Can you work these out from the model? Positions are in its coordinate system, mm. Face numbers are marked on the shaded views. A direction names the side the tool comes from. Round coordinates to 2 decimals unless told otherwise and drop trailing zeros. Order: outer loops, then holes, each group sorted by start corner. A loop starts at its lowest first (then second) coordinate and runs counter-clockwise, first axis right, second up. Notation, with made-up numbers: M -21.75,44.25 L 10.25,44.25 A16 cw 10.25,48.25 Z; hole C 37,44 d7. An arc over 180 degrees is marked long. Answer as a JSON object with one key per item and string values. Group by question number.
from build123d import *

# Parameters (mm, degrees)
BOX013_W                   = 14
BOX013_H                   = 3
BOX013_DEPTH               = 18
CYLINDER006_R              = 3.5
CYLINDER006_DEPTH          = 8
CYLINDER006_ROLL_ANGLE     = -90
CYLINDER_R                 = 0.6
CYLINDER_DEPTH             = 11
PRISM_DEPTH                = 10
PRISM_ROLL_ANGLE           = 90.00003
PRISM_PITCH_ANGLE          = -30.000033
PRISM_PLACEMENT_ANGLE      = -8e-06
BOX001_W                   = 10
BOX001_H                   = 18
BOX001_DEPTH               = 20
BOX002_W                   = 10
BOX002_H                   = 11
BOX002_DEPTH               = 15
BOX003_W                   = 10
BOX003_H                   = 25
BOX003_DEPTH               = 12
BOX004_W                   = 8.5
BOX004_H                   = 4
BOX004_DEPTH               = 7
BOX005_W                   = 8
BOX005_H                   = 4
BOX005_DEPTH               = 10.5
BOX006_W                   = 8.5
BOX006_H                   = 4
BOX006_DEPTH               = 7
BOX007_W                   = 13
BOX007_H                   = 4
BOX007_DEPTH               = 8
BOX008_W                   = 10
BOX008_H                   = 8.5
BOX008_DEPTH               = 8
BOX009_W                   = 5
BOX009_H                   = 14
BOX009_DEPTH               = 9
BOX010_W                   = 43
BOX010_H                   = 4
BOX010_DEPTH               = 19
SKETCH075_R                = 1.4
EXTRUDE_DEPTH              = 12
BOX011_W                   = 14
BOX011_H                   = 4
BOX011_DEPTH               = 12
BOX_W                      = 10
BOX_H                      = 56.75
BOX_DEPTH                  = 12
EXTRUDE073_DEPTH           = 25
EXTRUDE072_DEPTH           = 25
SKETCH072_R                = 4
SKETCH072_R_2              = 1.4
SKETCH072_R_3              = 2.25
EXTRUDE071_DEPTH           = 22.4
BOX012_W                   = 13
BOX012_H                   = 3
BOX012_DEPTH               = 15
EXTRUDE080_DEPTH           = 2.5
SKETCH071_W                = 47
SKETCH071_H                = 15
EXTRUDE070_DEPTH           = 2
EXTRUDE070_ROLL_ANGLE      = -0.000172
EXTRUDE070_PITCH_ANGLE     = -0.040176
EXTRUDE070_PLACEMENT_ANGLE = 2.8e-05


with BuildPart() as cube013:
    # Box013 → Box013 (new body)
    with BuildSketch(Plane(origin=(8, -54.5, 7), x_dir=(1, 0, 0), z_dir=(0, 0, 1))):
        with Locations((7, 1.5)):
            Rectangle(BOX013_W, BOX013_H)
    extrude(amount=BOX013_DEPTH)


with BuildPart() as cylinder006:
    # Cylinder006 → Cylinder006 (new body)
    with BuildSketch(Plane.XY):
        Circle(CYLINDER006_R)
    extrude(amount=CYLINDER006_DEPTH)


with BuildPart() as cylinder006_1:
    # Cylinder006 roll: moved
    add(cylinder006.part.rotate(Axis((0, 0, 0), (1, 0, 0)), CYLINDER006_ROLL_ANGLE))


with BuildPart() as cylinder006_2:
    # Cylinder006 placement: moved
    add(cylinder006_1.part.moved(Location((42.4, 48, 10))))


with BuildPart() as cylinder:
    # Cylinder → Cylinder (new body)
    with BuildSketch(Plane(origin=(46.125, 51.85, 17), x_dir=(1, 0, 0), z_dir=(0, 0, 1))):
        Circle(CYLINDER_R)
    extrude(amount=CYLINDER_DEPTH)


with BuildPart() as fusion032:
    # Prism → Prism (new body)
    with BuildSketch(Plane.XY):
        Polygon((5, 0), (2.5, 4.330127), (-2.5, 4.330127), (-5, 0), (-2.5, -4.330127), (2.5, -4.330127), align=None)
    extrude(amount=PRISM_DEPTH)


with BuildPart() as fusion032_1:
    # Prism roll: moved
    add(fusion032.part.rotate(Axis((0, 0, 0), (1, 0, 0)), PRISM_ROLL_ANGLE))


with BuildPart() as fusion032_2:
    # Prism pitch: moved
    add(fusion032_1.part.rotate(Axis((0, 0, 0), (0, 1, 0)), PRISM_PITCH_ANGLE))


with BuildPart() as fusion032_3:
    # Prism placement: moved
    add(fusion032_2.part.moved(Location((42.4, 51.75, 10))).rotate(Axis((42.4, 51.75, 10), (0, 0, 1)), PRISM_PLACEMENT_ANGLE))

    # Fusion032: union Cylinder006, Cylinder
    add(cylinder006_2.part)
    add(cylinder.part)


with BuildPart() as cube001:
    # Box001 → Box001 (new body)
    with BuildSketch(Plane(origin=(-67, 15.5, 8.5), x_dir=(1, 0, 0), z_dir=(0, 0, 1))):
        with Locations((5, 9)):
            Rectangle(BOX001_W, BOX001_H)
    extrude(amount=BOX001_DEPTH)


with BuildPart() as cube002:
    # Box002 → Box002 (new body)
    with BuildSketch(Plane(origin=(54, -25, 12), x_dir=(1, 0, 0), z_dir=(0, 0, 1))):
        with Locations((5, 5.5)):
            Rectangle(BOX002_W, BOX002_H)
    extrude(amount=BOX002_DEPTH)


with BuildPart() as cube003:
    # Box003 → Box003 (new body)
    with BuildSketch(Plane(origin=(54, -14, 15), x_dir=(1, 0, 0), z_dir=(0, 0, 1))):
        with Locations((5, 12.5)):
            Rectangle(BOX003_W, BOX003_H)
    extrude(amount=BOX003_DEPTH)


with BuildPart() as cube004:
    # Box004 → Box004 (new body)
    with BuildSketch(Plane(origin=(32.75, 51, 20), x_dir=(1, 0, 0), z_dir=(0, 0, 1))):
        with Locations((4.25, 2)):
            Rectangle(BOX004_W, BOX004_H)
    extrude(amount=BOX004_DEPTH)


with BuildPart() as cube005:
    # Box005 → Box005 (new body)
    with BuildSketch(Plane(origin=(19, 51, 16.5), x_dir=(1, 0, 0), z_dir=(0, 0, 1))):
        with Locations((4, 2)):
            Rectangle(BOX005_W, BOX005_H)
    extrude(amount=BOX005_DEPTH)


with BuildPart() as cube006:
    # Box006 → Box006 (new body)
    with BuildSketch(Plane(origin=(-45.9, 51, 20), x_dir=(1, 0, 0), z_dir=(0, 0, 1))):
        with Locations((4.25, 2)):
            Rectangle(BOX006_W, BOX006_H)
    extrude(amount=BOX006_DEPTH)


with BuildPart() as cube007:
    # Box007 → Box007 (new body)
    with BuildSketch(Plane(origin=(0.75, 51, 19.5), x_dir=(1, 0, 0), z_dir=(0, 0, 1))):
        with Locations((6.5, 2)):
            Rectangle(BOX007_W, BOX007_H)
    extrude(amount=BOX007_DEPTH)


with BuildPart() as cube008:
    # Box008 → Box008 (new body)
    with BuildSketch(Plane(origin=(54, 26.5, 20), x_dir=(1, 0, 0), z_dir=(0, 0, 1))):
        with Locations((5, 4.25)):
            Rectangle(BOX008_W, BOX008_H)
    extrude(amount=BOX008_DEPTH)


with BuildPart() as cube009:
    # Box009 → Box009 (new body)
    with BuildSketch(Plane(origin=(57, 23.75, 18.25), x_dir=(1, 0, 0), z_dir=(0, 0, 1))):
        with Locations((2.5, 7)):
            Rectangle(BOX009_W, BOX009_H)
    extrude(amount=BOX009_DEPTH)


with BuildPart() as cube010:
    # Box010 → Box010 (new body)
    with BuildSketch(Plane(origin=(-35, -56, 8), x_dir=(1, 0, 0), z_dir=(0, 0, 1))):
        with Locations((21.5, 2)):
            Rectangle(BOX010_W, BOX010_H)
    extrude(amount=BOX010_DEPTH)


with BuildPart() as extrude_body:
    # Sketch075 → Extrude (new body)
    with BuildSketch(Plane.XY.offset(27)):
        with Locations((-60, 46.5)):
            Circle(SKETCH075_R)
        with Locations((57.75, 46.5)):
            Circle(SKETCH075_R)
        with Locations((-60, -46.5)):
            Circle(SKETCH075_R)
        with Locations((57.75, -46.5)):
            Circle(SKETCH075_R)
    extrude(amount=-EXTRUDE_DEPTH)


with BuildPart() as cube011:
    # Box011 → Box011 (new body)
    with BuildSketch(Plane(origin=(8, -55, 15), x_dir=(1, 0, 0), z_dir=(0, 0, 1))):
        with Locations((7, 2)):
            Rectangle(BOX011_W, BOX011_H)
    extrude(amount=BOX011_DEPTH)


with BuildPart() as fusion:
    # Box → Box (new body)
    with BuildSketch(Plane(origin=(-67, -44, 15), x_dir=(1, 0, 0), z_dir=(0, 0, 1))):
        with Locations((5, 28.375)):
            Rectangle(BOX_W, BOX_H)
    extrude(amount=BOX_DEPTH)

    # Fusion: union Cube001, Cube002, Cube003, Cube004, Cube005, Cube006, Cube007, Cube008, Cube009, Cube010, Extrude body, Cube011
    add(cube001.part)
    add(cube002.part)
    add(cube003.part)
    add(cube004.part)
    add(cube005.part)
    add(cube006.part)
    add(cube007.part)
    add(cube008.part)
    add(cube009.part)
    add(cube010.part)
    add(extrude_body.part)
    add(cube011.part)


with BuildPart() as extrude073:
    # Sketch074 → Extrude073 (new body)
    with BuildSketch(Plane.XY):
        Polygon((53.5, -52.25), (-56.5, -52.25), (-57.5, -51.25), (-57.5, 50.75), (-56.5, 51.75), (53.5, 51.75), (55, 50.25), (55, -50.75), align=None)
    extrude(amount=EXTRUDE073_DEPTH)


with BuildPart() as cut001:
    # Sketch073 → Extrude072 (new body)
    with BuildSketch(Plane.XY):
        Polygon((54.25, -54.5), (-57.25, -54.5), (-65.25, -46.5), (-65.25, 46), (-57.25, 54), (54.25, 54), (61.25, 47), (61.25, -47.5), align=None)
    extrude(amount=EXTRUDE072_DEPTH)

    # Cut: cut Extrude073
    add(extrude073.part, mode=Mode.SUBTRACT)


with BuildPart() as cut001_1:
    # Cut placement: moved
    add(cut001.part.moved(Location((0, 0, 2))))

    # Cut001: cut Fusion
    add(fusion.part, mode=Mode.SUBTRACT)


with BuildPart() as extrude071:
    # Sketch072 → Extrude071 (new body)
    with BuildSketch(Plane.XY):
        with Locations((25.25, -42.25)):
            Circle(SKETCH072_R)
        with Locations((25.25, -42.25)):
            Circle(SKETCH072_R_2, mode=Mode.SUBTRACT)
        with Locations((53.25, -51.25)):
            Circle(SKETCH072_R_3)
        with BuildLine():
            Line((-53.75, 52.75), (-46.75, 52.75))
            Line((-46.75, 52.75), (-46.75, 47.25))
            ThreePointArc((-53.75, 47.25), (-50.25, 43.75), (-46.75, 47.25))
            Line((-53.75, 47.25), (-53.75, 52.75))
        make_face()
        with Locations((-50.25, 47.25)):
            Circle(SKETCH072_R_2, mode=Mode.SUBTRACT)
        with BuildLine():
            Line((46.75, 52.75), (53.75, 52.75))
            Line((53.75, 52.75), (53.75, 47.25))
            ThreePointArc((46.75, 47.25), (50.25, 43.75), (53.75, 47.25))
            Line((46.75, 47.25), (46.75, 52.75))
        make_face()
        with Locations((50.25, 47.25)):
            Circle(SKETCH072_R_2, mode=Mode.SUBTRACT)
        with BuildLine():
            Line((-53.75, -52.75), (-46.75, -52.75))
            Line((-46.75, -52.75), (-46.75, -47.25))
            ThreePointArc((-46.75, -47.25), (-50.25, -43.75), (-53.75, -47.25))
            Line((-53.75, -47.25), (-53.75, -52.75))
        make_face()
        with Locations((-50.25, -47.25)):
            Circle(SKETCH072_R_2, mode=Mode.SUBTRACT)
    extrude(amount=EXTRUDE071_DEPTH)


with BuildPart() as extrude071_1:
    # Extrude071 placement: moved
    add(extrude071.part.moved(Location((0, 0, 1))))


with BuildPart() as cube012:
    # Box012 → Box012 (new body)
    with BuildSketch(Plane(origin=(34, 48.75, 2), x_dir=(1, 0, 0), z_dir=(0, 0, 1))):
        with Locations((6.5, 1.5)):
            Rectangle(BOX012_W, BOX012_H)
    extrude(amount=BOX012_DEPTH)


with BuildPart() as extrude080:
    # Sketch091 → Extrude080 (new body)
    with BuildSketch(Plane.YZ):
        Polygon((0, 0), (0, 5), (-5, 5), (-2.5, 0), align=None)
    extrude(amount=EXTRUDE080_DEPTH)


with BuildPart() as extrude080_1:
    # Extrude080 placement: moved
    add(extrude080.part.moved(Location((43, 52, 16))))


with BuildPart() as cut005:
    # Sketch071 → Extrude070 (new body)
    with BuildSketch(Plane.XY):
        Polygon((54.25, -54.5), (-57.25, -54.5), (-65.25, -46.5), (-65.25, 46), (-57.25, 54), (54.25, 54), (61.25, 47), (61.25, -47.5), align=None)
        Polygon((-46.25, 42), (42.25, 42), (49.25, 35), (49.25, -16.5), (42.25, -23.5), (-46.25, -23.5), (-53.25, -16.5), (-53.25, 35), align=None, mode=Mode.SUBTRACT)
        with Locations((-13.25, -43)):
            Rectangle(SKETCH071_W, SKETCH071_H, mode=Mode.SUBTRACT)
    extrude(amount=EXTRUDE070_DEPTH)


with BuildPart() as cut005_1:
    # Extrude070 roll: moved
    add(cut005.part.rotate(Axis((0, 0, 0), (1, 0, 0)), EXTRUDE070_ROLL_ANGLE))


with BuildPart() as cut005_2:
    # Extrude070 pitch: moved
    add(cut005_1.part.rotate(Axis((0, 0, 0), (0, 1, 0)), EXTRUDE070_PITCH_ANGLE))


with BuildPart() as cut005_3:
    # Extrude070 placement: moved
    add(cut005_2.part.rotate(Axis((0, 0, 0), (0, 0, 1)), EXTRUDE070_PLACEMENT_ANGLE))

    # Fusion027: union Extrude071, Cube012, Extrude080
    add(extrude071_1.part)
    add(cube012.part)
    add(extrude080_1.part)

    # Fusion028: union Cut001
    add(cut001_1.part)

    # Cut003: cut Fusion032
    add(fusion032_3.part, mode=Mode.SUBTRACT)

    # Cut005: cut Cube013
    add(cube013.part, mode=Mode.SUBTRACT)


solid = cut005_3.part
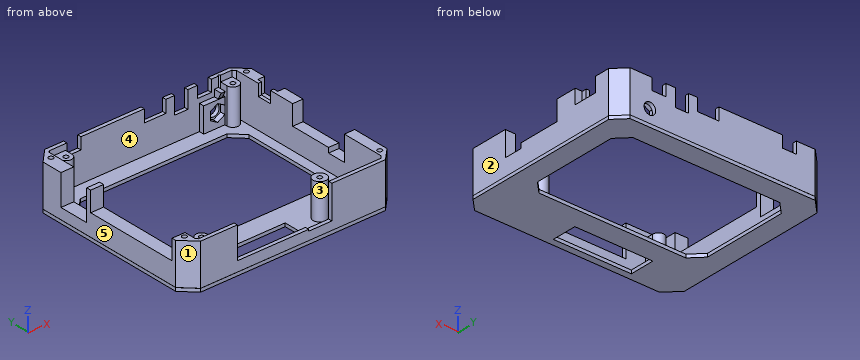
Item 1: I need wall thicknesses on line 1 (Y direction, x = -50.25, z = 15.75); line 2 (Y direction, x = 50.25, z = 16.25); line 3 (Y direction, x = -45.5, z = 6.5). Which ranges of each line are inside material? Lowest first, please.
Item 2: Suppose I cut it at D-D, the plane x = -60. Write out the boundary of the cut face in (y, z).
Item 3: On a 3-axis mill with a long thin cutter (end or side, diameter ignored), from which of +Z, -Z, +X, -X, +Y, -Y can I reach the whole of each face in a straight line? I mean the marked faces 4 and 5. Say none if no direction works.
Item 4: If we mould it in two halves opening along X, with no side actions, what happens to the marked faces 1, 2 and 3? For each: +X half, -X half, draft (parallel to the pull), parting line (faces both ways), or undercut.
Item 5: Suppose I cut it at B-B, the plane x = 4.5. State how many separate pieces and enclosed holes the cut face has, and give its area (3 significant figures).
Item 6: I'm going to push flat-ended pins straight in: pin 1 Ø1.6 at (x, z) = (56, 23.5) entering from -Y; pin 2 Ø6 at (x, y) = (44, 6.5) entering from -Z; pin 3 Ø0.7 at (x, y) = (-21, -54) entering from +Z; pin 4 Ø5 at (y, z) = (50.5, 11) entering from -X. Where does each tip first touch, or does it pass through?
Computed:
{
 "1": {"line 1": "y = -54.5 to -48.65, -45.85 to -43.75, 43.75 to 45.85, 48.65 to 54", "line 2": "y = -54.5 to -52.25, 43.75 to 45.85, 48.65 to 54", "line 3": "y = -54.5 to -52.25, 51.75 to 54"},
 "2": {"outline": "M -51.75,-0.04 L 51.25,-0.04 L 51.25,1.96 L -51.75,1.96 Z; M -51.75,2 L 51.25,2 L 51.25,27 L 47.9,27 L 47.9,15 L 45.1,15 L 45.1,27 L 33.5,27 L 33.5,8.5 L 15.5,8.5 L 15.5,27 L 12.75,27 L 12.75,15 L -44,15 L -44,27 L -45.1,27 L -45.1,15 L -47.9,15 L -47.9,27 L -51.75,27 Z"},
 "3": {"face 4": "+Z", "face 5": "+Z, -Z, -X, +Y, -Y"},
 "4": {"face 1": "-X half", "face 2": "+X half", "face 3": "undercut"},
 "5": {"separate pieces": "3", "enclosed holes": "0", "area": "109 mm^2"},
 "6": {"pin 1": "stops at y = -53.55", "pin 2": "passes through", "pin 3": "stops at z = 8", "pin 4": "stops at x = -63.25"}
}
